Check sheet for the modelled part. Datum: model origin and axes. Units: mm. A direction names the side the tool comes from. Round coordinates to 2 decimals unless told otherwise and drop trailing zeros. Write each loop counter-clockwise with the first axis right and the second up, starting at its lowest first coordinate (ties: lowest second). Pieces come first, ordered by that corner, then holes.
Item 1: Release check for a two-part mould opening along Z. For faces 1 (the cylindrical face through (-0.035, 15.276, 6.033)), 2 (the flat face through (0, -17.78, 3)), 3 (the flat face through (0, 0, 83.82)) record: pulls with the +Z half, pulls with the -Z half, needs draft (parallel to the pull), parting line crosses it, or undercut.
Item 2: Section check D-D, the plane x = -0.75. Record the cut outline in (y, z), plus the area to 3 significant figures.
Item 3: Depth check by flat-ended pin: pin 1 (3 mm diameter, centred on x = 1, y = -7.5, fed in from -Z); pin 2 (5 mm diameter, centred on x = 1, z = 49.5, fed in from -Y). Enter the tip coordinate at first touch or a pass-through.
Item 4: Material ranges on line 1 along Y through (x, z) = (0, 2.55); line 2 along Z through (x, y) = (-2, 2.5); line 3 along X through (y, z) = (16, 8.5), recorded low to high.
Item 5: Section check A-A, the plane z = 11. Record the cut outline in (x, y).
Item 6: Set-up check for faces 4 (the flat face through (0, -3, 78.74)), 5 (the flat face through (1.588, 15, 41)), 6 (the flat face through (2, 17.78, 41)): record each of +Z, -Z, +X, -X, +Y, -Y from which the full face is reachable in a straight line by a thin tool's end or side.
Item 7: Section check C-C, the plane y = -15.24. Record the cut outline in (x, z), plus the area to 3 significant figures.
Item 8: Section check B-B, the plane y = 10. Record the cut outline in (x, z), plus the area to 3 significant figures.
from build123d import *

# Parameters (mm, degrees)
SKETCH1_W           = 9.525
SKETCH1_H           = 35.56
BOSS_EXTRUDE1_DEPTH = 83.82
SKETCH2_W           = 73.66
SKETCH2_H           = 30.48
CUT_EXTRUDE1_DEPTH  = 78.74
CUT_EXTRUDE2_DEPTH  = 78.74
SKETCH4_R           = 1.5875
CUT_EXTRUDE3_DEPTH  = 84.82
SKETCH5_R           = 1.5875
CUT_EXTRUDE4_DEPTH  = 84.82


with BuildPart() as part:
    # Sketch1 → Boss-Extrude1 (new body)
    with BuildSketch(Plane.XY):
        Rectangle(SKETCH1_W, SKETCH1_H)
    extrude(amount=BOSS_EXTRUDE1_DEPTH)

    # Sketch2 → Cut-Extrude1 (cut)
    with BuildSketch(Plane(origin=(4.7625, 0, 0), x_dir=(0, 0, -1), z_dir=(1, 0, 0))):
        with Locations((-41.91, -2.54)):
            Rectangle(SKETCH2_W, SKETCH2_H)
    extrude(amount=-CUT_EXTRUDE1_DEPTH, mode=Mode.SUBTRACT)

    # Sketch3 → Cut-Extrude2 (cut)
    with BuildSketch(Plane(origin=(0, 17.78, 0), x_dir=(1, 0, 0), z_dir=(0, 1, 0))):
        with BuildLine():
            Line((-1.5875, -76.2), (-1.5875, -7.62))
            ThreePointArc((-1.5875, -7.62), (0, -6.0325), (1.5875, -7.62))
            Line((1.5875, -7.62), (1.5875, -76.2))
            ThreePointArc((1.5875, -76.2), (0, -77.7875), (-1.5875, -76.2))
        make_face()
    extrude(amount=-CUT_EXTRUDE2_DEPTH, mode=Mode.SUBTRACT)

    # Sketch4 → Cut-Extrude3 (cut, through all)
    with BuildSketch(Plane.XY.offset(83.82)):
        with Locations((0, -15.24)):
            Circle(SKETCH4_R)
    extrude(amount=-CUT_EXTRUDE3_DEPTH, mode=Mode.SUBTRACT)

    # Sketch5 → Cut-Extrude4 (cut, through all)
    with BuildSketch(Plane.XY.offset(83.82)):
        with Locations((0, 6.35)):
            Circle(SKETCH5_R)
    extrude(amount=-CUT_EXTRUDE4_DEPTH, mode=Mode.SUBTRACT)


solid = part.part
Values found:
1. face 1: undercut
1. face 2: needs draft
1. face 3: pulls with the +Z half
2. outline: (-17.78, 0) - (-16.64, 0) - (-16.64, 5.08) - (-17.78, 5.08) - close; (-17.78, 78.74) - (-16.64, 78.74) - (-16.64, 83.82) - (-17.78, 83.82) - close; (-13.84, 0) - (4.95, 0) - (4.95, 5.08) - (-13.84, 5.08) - close; (-13.84, 78.74) - (4.95, 78.74) - (4.95, 83.82) - (-13.84, 83.82) - close; (7.75, 0) - (17.78, 0) - (17.78, 6.22) - (12.7, 6.22) - (12.7, 5.08) - (7.75, 5.08) - close; (7.75, 78.74) - (12.7, 78.74) - (12.7, 77.6) - (17.78, 77.6) - (17.78, 83.82) - (7.75, 83.82) - close
2. area: 316 mm2
3. pin 1: stops at z = 0
3. pin 2: stops at y = 12.7
4. line 1: y = -17.78 to -16.83, -13.65 to 4.76, 7.94 to 17.78
4. line 2: z = 0 to 5.08, 78.74 to 83.82
4. line 3: x = -4.76 to -1.59, 1.59 to 4.76
5. outline: (-4.76, 12.7) - (-1.59, 12.7) - (-1.59, 17.78) - (-4.76, 17.78) - close; (1.59, 12.7) - (4.76, 12.7) - (4.76, 17.78) - (1.59, 17.78) - close
6. face 4: +X, -X, -Y
6. face 5: +Y, -Y
6. face 6: +Z, -Z, +X, -X, +Y
7. outline: (-4.76, 0) - (-1.59, 0) - (-1.59, 5.08) - (-4.76, 5.08) - close; (-4.76, 78.74) - (-1.59, 78.74) - (-1.59, 83.82) - (-4.76, 83.82) - close; (1.59, 0) - (4.76, 0) - (4.76, 5.08) - (1.59, 5.08) - close; (1.59, 78.74) - (4.76, 78.74) - (4.76, 83.82) - (1.59, 83.82) - close
7. area: 64.5 mm2
8. outline: (-4.76, 0) - (4.76, 0) - (4.76, 5.08) - (-4.76, 5.08) - close; (-4.76, 78.74) - (4.76, 78.74) - (4.76, 83.82) - (-4.76, 83.82) - close
8. area: 96.8 mm2
